Here's how the part is built. I have some questions about the finished solid (model axes, mm). Face numbers are marked on the shaded views. A direction names the side the tool comes from. Coordinates: 2 decimals unless noted, no trailing zeros. Write each loop counter-clockwise with the first axis right and the second up, starting at its lowest first coordinate (ties: lowest second). Pieces come first, ordered by that corner, then holes. Notation, with made-up numbers: (-19.5, 60) -> (4.5, 60) arc R30 cw to (4.5, 96) -> close; hole circle Ø7 at (62.5, -4). An arc over 180 degrees is marked (long way). Use a Markdown table: item, result. Add a question column.
Item 1: Imagine slicing it at D-D, the plane x = -40. Write out the boundary of the cut face in (y, z), and give its area (3 significant figures).
Item 2: Will these pins go through, and if not, where does the flat tip stop? pin 1 Ø3 at (x, z) = (31.5, 23) entering from +Y; pin 2 Ø2 at (x, y) = (-4, 166.5) entering from +Z; pin 3 Ø8 at (x, y) = (-2, 105.5) entering from -Z.
Item 3: If I drill on line 1 along Y through (x, z) = (-28, 0); line 2 along X through (y, z) = (30, -8.5); line 3 along Y through (x, z) = (-18, -82), over which ranges is the centre line in solid material (lowest first)? Write a range as from..to.
Item 4: Imagine slicing it at C-C, the plane z = 25. Write out the boundary of the cut face in (x, y).
Item 5: Imagine slicing it at A-A, the plane x = 0. Write out the boundary of the cut face in (y, z).
Item 6: Imagine slicing it at B-B, the plane y = 142. Write out the boundary of the cut face in (x, z), and give its area (3 significant figures).
Item 7: On a 3-axis mill with a long thin cutter (end or side, diameter ignored), from which of +Z, -Z, +X, -X, +Y, -Y can I reach the whole of each face in a straight line? I mean the marked faces 1, 2 and 3. Say none if no direction works.
```python
from build123d import *

# Parameters (mm, degrees)
SKETCH1_R                = 30
BOSS_EXTRUDE1_DEPTH      = 120
BOSS_EXTRUDE2_DEPTH      = 40
BOSS_EXTRUDE2_DEPTH_BACK = 20
SKETCH2_R                = 50
SKETCH3_R                = 20
BOSS_EXTRUDE3_DEPTH      = 300


with BuildPart() as part:
    # Sketch1 → Boss-Extrude1 (new body)
    with BuildSketch(Plane.XY):
        Circle(SKETCH1_R)
    extrude(amount=-BOSS_EXTRUDE1_DEPTH)

    # Sketch2 → Boss-Extrude2 (add, two sides: drawn at the far end of the back side and taken through both)
    with BuildSketch(Plane(origin=(0, 0, 0), x_dir=(1, 0, 0), z_dir=(0, 1, 0)).offset(-BOSS_EXTRUDE2_DEPTH_BACK)):
        with Locations(Location((0, 0, 0), (0, 0, 270))):
            Circle(SKETCH2_R)
    extrude(amount=BOSS_EXTRUDE2_DEPTH + BOSS_EXTRUDE2_DEPTH_BACK)

    # Sketch3 → Boss-Extrude3 (add)
    with BuildSketch(Plane(origin=(0, 40, 0), x_dir=(1, 0, 0), z_dir=(0, 1, 0))):
        with Locations(Location((0, 0, 0), (0, 0, 270))):
            Circle(SKETCH3_R)
    extrude(amount=BOSS_EXTRUDE3_DEPTH)


solid = part.part
```
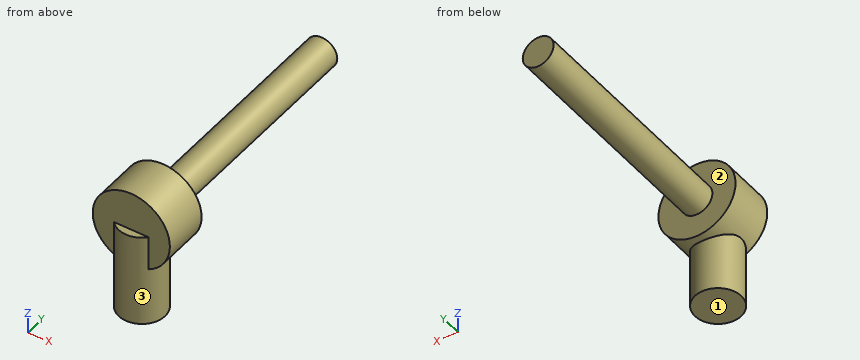
Ans:
| question | item | result |
|---|---|---|
| 1 | outline | (-20, -30) -> (40, -30) -> (40, 30) -> (-20, 30) -> close |
| 1 | area | 3,600 mm^2 |
| 2 | pin 1 | stops at y = 40 |
| 2 | pin 2 | stops at z = 19.77 |
| 2 | pin 3 | stops at z = -20 |
| 3 | line 1 | y = -20..40 |
| 3 | line 2 | x = -49.27..49.27 |
| 3 | line 3 | y = -24..24 |
| 4 | outline | (-43.3, -20) -> (43.3, -20) -> (43.3, 40) -> (-43.3, 40) -> close |
| 5 | outline | (-30, -120) -> (30, -120) -> (30, -50) -> (40, -50) -> (40, -20) -> (340, -20) -> (340, 20) -> (40, 20) -> (40, 50) -> (-20, 50) -> (-20, 0) -> (-30, 0) -> close |
| 6 | outline | circle Ø40 at (0, 0) |
| 6 | area | 1,260 mm^2 |
| 7 | face 1 | -Z, +X, -X, +Y, -Y |
| 7 | face 2 | +Y |
| 7 | face 3 | -Z |
